For this review, use the dimensioned drawing (mm, ordinates from the lowest corner) and the shaded views. A direction names the side the tool comes from. Round coordinates to 2 decimals unless told otherwise and drop trailing zeros. Write each loop counter-clockwise with the first axis right and the second up, starting at its lowest first coordinate (ties: lowest second). Pieces come first, ordered by that corner, then holes.
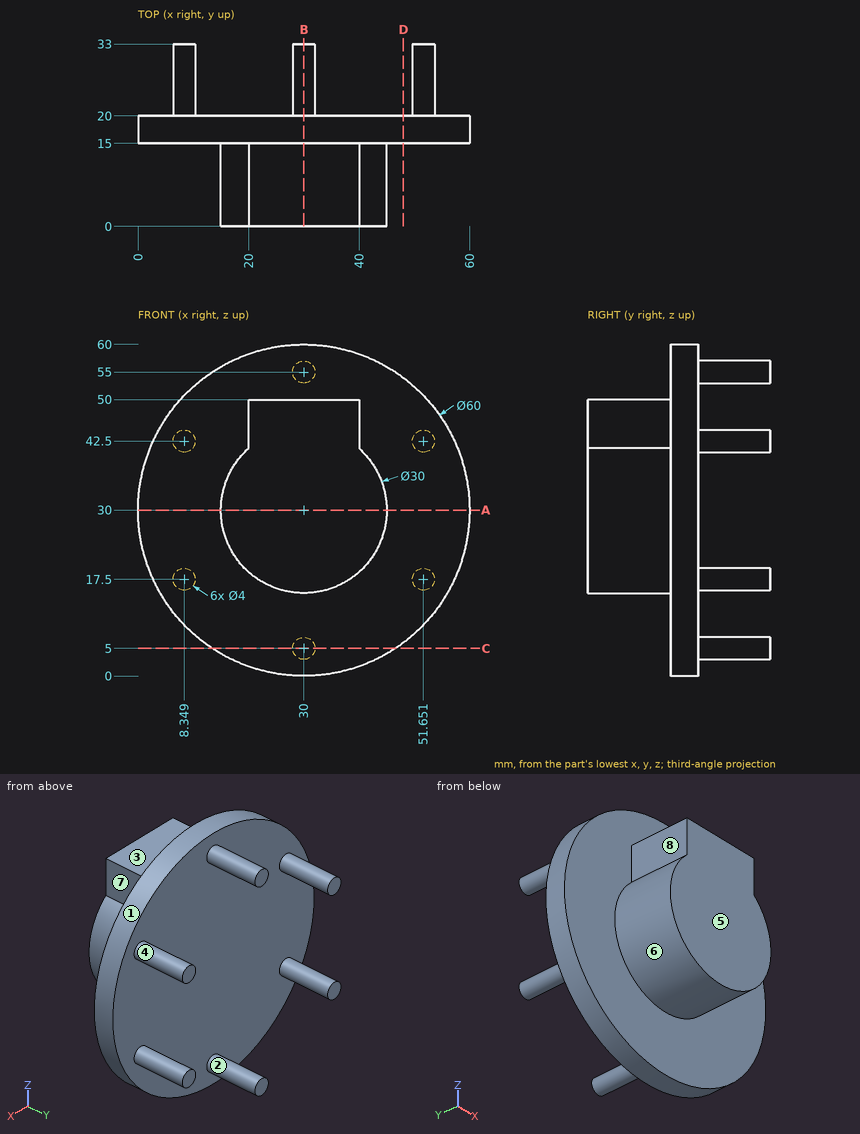
(1) We need section D-D, the plane x = 48. Give the boundary of the cut face in (y, z), and give its area (3 significant figures).
Geometry check:
outline: (15, 6) - (20, 6) - (20, 54) - (15, 54) - close
area: 240 mm2
(2) For pin 1 Ø2.5 at (y, z) = (7.5, 44.5) entering from +X; pin 2 Ø6 at (x, z) = (39, 51) entering from +Y; pin 3 Ø1 at (x, y) = (19.5, 17) entering from +Z (1 decimal); pin 4 Ø12 at (x, z) = (15, 42) entering from +Y, all flat-tipped, find the tip position at first contact; note any pin that passes through.
Geometry check:
pin 1: stops at x = 40
pin 2: stops at y = 20
pin 3: stops at z = 58.3
pin 4: stops at y = 33
(3) We need section B-B, the plane x = 30. Give the boundary of the cut face in (y, z).
Geometry check:
outline: (0, 15) - (15, 15) - (15, 0) - (20, 0) - (20, 3) - (33, 3) - (33, 7) - (20, 7) - (20, 53) - (33, 53) - (33, 57) - (20, 57) - (20, 60) - (15, 60) - (15, 50) - (0, 50) - close
(4) Mouldability with a two-part tool opening along Z and no side actions: class the marked faces 1, 2 and 3 as pulls with the +Z half, pulls with the -Z half, needs draft (parallel to the pull), parting line crosses it, or undercut.
Geometry check:
face 1: parting line crosses it
face 2: undercut
face 3: pulls with the +Z half
(5) For line 1 along Y through (x, z) = (26, 7.5); line 2 along Y through (x, z) = (27, 22.5); line 3 along X through (y, z) = (16, 19), list the stretches that pass through material, from the lowest coordinate up.
Geometry check:
line 1: y = 15 to 20
line 2: y = 0 to 20
line 3: x = 2.09 to 57.91
(6) We need section C-C, the plane z = 5. Give the boundary of the cut face in (x, y), and give its area (3 significant figures).
Geometry check:
outline: (13.42, 15) - (46.58, 15) - (46.58, 20) - (32, 20) - (32, 33) - (28, 33) - (28, 20) - (13.42, 20) - close
area: 218 mm2
(7) We need section A-A, the plane z = 30. Give the boundary of the cut face in (x, y), and give its area (3 significant figures).
Geometry check:
outline: (0, 15) - (15, 15) - (15, 0) - (45, 0) - (45, 15) - (60, 15) - (60, 20) - (0, 20) - close
area: 750 mm2
(8) For the marked faces 4, 5, 6, 7 and 8, list the 3-axis set-ups (+Z, -Z, +X, -X, +Y, -Y) from which the entire face can be reached by the end or side of a thin tool; tool diameter is ignored.
Geometry check:
face 4: +Y
face 5: +Z, -Z, +X, -X, -Y
face 6: -Y
face 7: +Z, +X, -Y
face 8: +Z, -X, -Y
